Work out the finished part from the listing and answer in its coordinate system (mm). A direction names the side the tool comes from. Coordinates: 2 decimals unless noted, no trailing zeros. Loops run counter-clockwise (first coordinate to the right, second up) from the corner with the lowest first, then second, coordinate; pieces in that order, holes last. Notation, with made-up numbers: (24.25, -23.75) - (79.25, -23.75) arc R14 cw to (79.25, -8.75) - close; hole circle Ø2 at (-28, 51). An arc over 180 degrees is marked (long way). Write each question's results on one line, items separated by ' | '. Start each with the question number.
1. Which of the six approach directions +Z, -Z, +X, -X, +Y, -Y give full straight-line access (tool end or side, diameter ignored) to faces 1 (the flat face through (-15.24, 52, 0)), 2 (the cylindrical face through (-13.886, 29.344, -3.083)), 3 (the flat face through (0, 52, 0)), 4 (the flat face through (0, -22.86, 0)), 5 (the flat face through (-8, 52, 7.62))?
2. A cutting plane is placed at A-A on y = 39. Determine the outline of the cut face in (x, z).
3. A cutting plane is placed at B-B on y = 23. Determine the outline of the cut face in (x, z), then the cut area to 3 significant figures.
4. Find the intervals of material crossed by line 1 along Y through (x, z) = (-4, 2.5); line 2 along Y through (x, z) = (18.5, 10); line 3 along Z through (x, y) = (5, 18.5), in increasing order. Write a range as [from, to].
5. Determine the mould class of faces 6 (the flat face through (-8, 52, -7.62)), 7 (the flat face through (-8, 56.261, 0)), 8 (the flat face through (0, 33.401, -11)), 9 (the cylindrical face through (4.037, 40.914, -9.737)) for opening direction Y: released by +Y, released by -Y, zero draft, split by the parting line, or undercut.
6. Each of these flat-tipped pins is pushed along its axis until it touches: P1, Ø2, axis at x = 7, y = 35, coming from the -Z side; P2, Ø6, axis at y = 52, z = -1.5, coming from the +X side; P3, Ø5, axis at y = 42.5, z = 8, coming from the -X side. Where does it stop, or does it pass through?
from build123d import *

# Parameters (mm, degrees)
SKETCH1_R           = 21.971
BOSS_EXTRUDE1_DEPTH = 25.4
SKETCH2_R           = 14.224
BOSS_EXTRUDE2_DEPTH = 8.001
SKETCH3_R           = 10.541
BOSS_EXTRUDE3_DEPTH = 15.24
BOSS_EXTRUDE4_DEPTH = 7.62
SKETCH5_R           = 15.24
BOSS_EXTRUDE5_DEPTH = 22.86
FILLET1_R           = 12.7
FILLET2_R           = 12.7


with BuildPart() as part:
    # Sketch1 → Boss-Extrude1 (new body)
    with BuildSketch(Plane(origin=(0, 0, 0), x_dir=(1, 0, 0), z_dir=(0, 1, 0))):
        with Locations(Location((0, 0, 0), (0, 0, 270))):
            Circle(SKETCH1_R)
    extrude(amount=BOSS_EXTRUDE1_DEPTH)

    # Sketch2 → Boss-Extrude2 (add)
    with BuildSketch(Plane(origin=(0, 25.4, 0), x_dir=(1, 0, 0), z_dir=(0, 1, 0))):
        with Locations(Location((0, 0, 0), (0, 0, 270))):
            Circle(SKETCH2_R)
    extrude(amount=BOSS_EXTRUDE2_DEPTH)

    # Sketch3 → Boss-Extrude3 (add)
    with BuildSketch(Plane(origin=(0, 33.401, 0), x_dir=(1, 0, 0), z_dir=(0, 1, 0))):
        with Locations(Location((0, 0, 0), (0, 0, 90))):
            Circle(SKETCH3_R)
    extrude(amount=BOSS_EXTRUDE3_DEPTH)

    # Sketch4 → Boss-Extrude4 (add)
    with BuildSketch(Plane(origin=(0, 48.641, 0), x_dir=(1, 0, 0), z_dir=(0, 1, 0))):
        Polygon((0, 0), (0, 7.62), (-15.24, 7.62), (-15.24, 0), (-15.24, -7.62), (0, -7.62), align=None)
    extrude(amount=BOSS_EXTRUDE4_DEPTH)

    # Sketch5 → Boss-Extrude5 (add)
    with BuildSketch(Plane.XZ):
        with Locations(Location((0, 0, 0), (0, 0, 90))):
            Circle(SKETCH5_R)
    extrude(amount=BOSS_EXTRUDE5_DEPTH)

    # Fillet1
    # the kernel refuses this fillet: 12.7 mm, written as the material it adds along each edge
    with BuildSketch(Plane(origin=(0, 0, 0), x_dir=(0, 0, 1), z_dir=(1, 0, 0))) as fillet1_piece_1:
        with BuildLine():
            CenterArc((27.94, 11.209863469), FILLET1_R, 180, 61.965703465)
            Line((15.24, 11.209863469), (14.986, 11.209863469))
            Line((14.986, 11.209863469), (14.986, 0))
            Line((14.986, 0), (15.24, -0.254))
            ThreePointArc((15.24, -0.254), (18.6055, -0.254), (21.85162, -0.224197269))
            Line((21.85162, -0.224197269), (21.971, 0))
        make_face()
    revolve(axis=Axis((0, 0, 0), (0, -1, 0)))

    # Fillet2
    fillet2_edges = [part.edges().sort_by_distance(p)[0] for p in [
        (0, -22.86, -15.24),
    ]]
    fillet(fillet2_edges, radius=FILLET2_R)


solid = part.part
Values:
1) face 1: +Z, -Z, -X, +Y | face 2: none | face 3: +Z, -Z, +X, +Y | face 4: +Z, -Z, +X, -X, -Y | face 5: +Z, +X, -X, +Y
2) outline: circle Ø21.08 at (0, 0)
3) outline: circle Ø43.94 at (0, 0) | area: 1,520 mm^2
4) line 1: [-22.68, 56.26] | line 2: [-0.55, 25.4] | line 3: [-21.39, 21.39]
5) face 6: zero draft | face 7: released by +Y | face 8: undercut | face 9: undercut
6) P1: z = -8.67 | P2: x = 0 | P3: x = -8.99
